Autodesk Inventor part; units mm, degrees
ref_plane "YZ Plane" through (0, 0, 0) normal (1, 0, 0) x (0, 1, 0)
ref_plane "XZ Plane" through (0, 0, 0) normal (0, 1, 0) x (-1, 0, 0)
ref_plane "XY Plane" through (0, 0, 0) normal (0, 0, 1) x (1, 0, 0)
sketch "Sketch1" plane through (0, 0, 0) normal (0, 0, 1) x (1, 0, 0)
  line L0 (-11.5809, 11.3971) -> (-46.8809, 11.3971)
  line L1 (-46.8809, 11.3971) -> (-46.8809, 1.8971)
  line L2 (-46.8809, 1.8971) -> (-11.5809, 1.8971)
  line L3 (-11.5809, 1.8971) -> (-11.5809, 11.3971)
  line L4 (-46.8809, 6.6471) -> (-11.5809, 6.6471)
  line L5 (-11.5809, 6.6471) -> (-11.5809, 1.8971)
  line L6 (-11.5809, 4.2721) -> (-46.8809, 4.2721)
  line L7 (-46.8809, 4.2721) -> (-44.5059, 1.8971)
  line L8 (-46.8809, 4.2721) -> (-43.5221, 4.2721) construction
  line L9 (-44.5059, 1.8971) -> (-44.5059, 11.3971)
  line L10 (-11.5809, 4.2721) -> (-13.9559, 1.8971)
  line L11 (-13.9559, 11.3971) -> (-13.9559, 1.8971)
  point P0 (0, 0)
  dimension "d0" = 35.3
  dimension "d1" = 9.5
  dimension "d2" = 45
extrude "Extrusion1" add sketch "Sketch1" along normal blind 450 contours L3 L4 L11 L0 | L3 L6 L11 L4 | L9 L4 L1 L0 | L10 L11 L6 | L3 L2 L10 | L9 L6 L1 L4 | L11 L2 L9 L6 | L9 L7 L6 | L2 L1 L7
sketch "Sketch2" plane through (-44.5059, 4.2721, 0) normal (0, 1, 0) x (1, 0, 0)
  line L0 (30.55, 0) -> (0, 0)
  line L1 (0, -450) -> (30.55, -450)
  line L2 (15.275, 0) -> (15.275, -26)
  circle A0 centre (15.275, -26) radius 2.15
  line L3 (15.275, -26) -> (15.275, -410)
  line L4 (15.275, -26) -> (15.275, -378)
  circle A1 centre (15.275, -378) radius 2.15
  circle A2 centre (15.275, -410) radius 2.15
  point P0 (44.5059, 0)
  dimension "d5" = 26
  dimension "d6" = 4.3
  dimension "d7" = 384
  dimension "d8" = 352
extrude "Extrusion2" cut sketch "Sketch2" against normal blind 450
sketch "Sketch3" plane through (0, 0, 450) normal (0, 0, 1) x (1, 0, 0)
  line L0 (-11.5809, 1.8971) -> (-46.8809, 1.8971)
  line L1 (-11.5809, 11.3971) -> (-11.5809, 1.8971)
  line L2 (-13.9559, 11.3971) -> (-11.5809, 11.3971)
  line L3 (-13.9559, 4.2721) -> (-13.9559, 11.3971)
  line L4 (-44.5059, 4.2721) -> (-13.9559, 4.2721)
  line L5 (-44.5059, 11.3971) -> (-44.5059, 4.2721)
  line L6 (-46.8809, 11.3971) -> (-44.5059, 11.3971)
  line L7 (-46.8809, 1.8971) -> (-46.8809, 11.3971)
  point P0 (0, 0)
extrude "Extrusion3" cut sketch "Sketch3" against normal blind 419.1
sketch "Sketch4" plane through (0, 0, 0) normal (0, 0, -1) x (-1, 0, 0)
  line L0 (11.5809, 1.8971) -> (11.5809, 11.3971)
  line L1 (46.8809, 1.8971) -> (11.5809, 1.8971)
  line L2 (46.8809, 11.3971) -> (46.8809, 1.8971)
  line L3 (44.5059, 11.3971) -> (46.8809, 11.3971)
  line L4 (44.5059, 4.2721) -> (44.5059, 11.3971)
  line L5 (13.9559, 4.2721) -> (44.5059, 4.2721)
  line L6 (13.9559, 11.3971) -> (13.9559, 4.2721)
  line L7 (11.5809, 11.3971) -> (13.9559, 11.3971)
  point P0 (0, 0)
extrude "Extrusion4" add sketch "Sketch4" against normal blind 426.2437
sketch "Sketch5" plane through (-44.5059, 4.2721, 0) normal (0, 1, 0) x (1, 0, 0)
  line L0 (30.55, 0) -> (0, 0)
  line L1 (0, -426.2437) -> (30.55, -426.2437)
  line L2 (15.275, 0) -> (15.275, -63.246)
  circle A0 centre (15.275, -63.246) radius 2.3495
  line L3 (15.275, 0) -> (15.275, -203.2)
  line L4 (15.275, -203.2) -> (15.275, -200.8505)
  circle A1 centre (15.275, -200.8505) radius 2.3495
  line L5 (15.275, 0) -> (15.275, -419.1)
  circle A2 centre (15.275, -419.1) radius 2.3495
  point P0 (44.5059, 0)
  dimension "d15" = 63.246
  dimension "d16" = 4.699
  dimension "d17" = 203.2
  dimension "d18" = 2.3495
  dimension "d19" = 419.1
extrude "Extrusion5" cut sketch "Sketch5" against normal blind 426.2437
sketch "Sketch6" plane through (0, 0, 426.2437) normal (0, 0, 1) x (1, 0, 0)
  line L0 (-11.5809, 1.8971) -> (-46.8809, 1.8971)
  line L1 (-11.5809, 11.3971) -> (-11.5809, 1.8971)
  line L2 (-13.9559, 11.3971) -> (-11.5809, 11.3971)
  line L3 (-13.9559, 4.2721) -> (-13.9559, 11.3971)
  line L4 (-44.5059, 4.2721) -> (-13.9559, 4.2721)
  line L5 (-44.5059, 11.3971) -> (-44.5059, 4.2721)
  line L6 (-46.8809, 11.3971) -> (-44.5059, 11.3971)
  line L7 (-46.8809, 1.8971) -> (-46.8809, 11.3971)
  point P0 (0, 0)
extrude "Extrusion6" add sketch "Sketch6" along normal blind 0.7937
properties part number "1"
Check sheet for the modelled part. Datum: model origin and axes. Units: mm. A direction names the side the tool comes from. Coordinates: 2 decimals unless noted, no trailing zeros. Loops run counter-clockwise (first coordinate to the right, second up) from the corner with the lowest first, then second, coordinate; pieces in that order, holes last. Notation, with made-up numbers: M 15,-22.75 L 19,-22.75 A21 ccw 19,-16.75 Z; hole C -30,57 d4. An arc over 180 degrees is marked long. Answer as a JSON object with one key per item and string values.
1. Depth check by flat-ended pin: P1, Ø1.5, axis at x = -15, y = 9, coming from the +Z side; P2, Ø7.5, axis at x = -29.23, z = 200.85, coming from the +Y side. Enter the tip coordinate at first touch or a pass-through.
Outcome:
{"P1": "through", "P2": "y = 4.27"}
2. Sectioned sample at B-B on z = 376. Record the cut outline in (x, y), and give its area (3 significant figures).
Outcome:
{"outline": "M -46.88,1.9 L -11.58,1.9 L -11.58,11.4 L -13.96,11.4 L -13.96,4.27 L -44.51,4.27 L -44.51,11.4 L -46.88,11.4 Z", "area": "118 mm²"}
3. Access from +Z, -Z, +X, -X, +Y, -Y to the whole of each face (thin tool, end or side, straight path). Record for faces 4 (the flat face through (-29, 4, 0)), 5 (the flat face through (-44.506, 8, 211)).
Outcome:
{"face 4": "-Z, +X, -X, +Y, -Y", "face 5": "+Z, -Z, +Y"}
4. Release check for a two-part mould opening along X. For faces 1 (the flat face through (-29, 1.897, 211)), 2 (the flat face through (-46.881, 7, 211)), 3 (the flat face through (-13.956, 8, 211)) record: pulls with the +X half, pulls with the -X half, needs draft (parallel to the pull), parting line crosses it, or undercut.
Outcome:
{"face 1": "needs draft", "face 2": "pulls with the -X half", "face 3": "undercut"}
5. Scan lines: L1, parallel to X at y = 7.25, z = 338; L2, parallel to X at y = 2.8, z = 419.1; L3, parallel to Y at x = -22, z = 258. Record each from-to range of solid material in increasing order. Write a range as from..to.
Outcome:
{"L1": "-46.88..-44.51, -13.96..-11.58", "L2": "-46.88..-31.58, -26.88..-11.58", "L3": "1.9..4.27"}
6. Sectioned sample at C-C on x = -22. Record the cut outline in (y, z).
Outcome:
{"outline": "M 1.9,0 L 4.27,0 L 4.27,427.04 L 1.9,427.04 Z"}
7. Sectioned sample at A-A on y = 5.75. Record the cut outline in (x, z), and give its area (3 significant figures).
Outcome:
{"outline": "M -46.88,0 L -44.51,0 L -44.51,427.04 L -46.88,427.04 Z; M -13.96,0 L -11.58,0 L -11.58,427.04 L -13.96,427.04 Z", "area": "2,030 mm²"}
